Answer from the drawing. Dimensions are ordinates in mm from the lowest x, y and z of the part. A direction names the side the tool comes from. Round coordinates to 2 decimals unless told otherwise and drop trailing zeros. Loops run counter-clockwise (first coordinate to the right, second up) from the corner with the lowest first, then second, coordinate; pieces in that order, holes last. Notation, with made-up numbers: (81.5, 4.5) - (93.5, 4.5) arc R3 cw to (93.5, 9.5) - close; hole circle Ø5 at (50, 0.25). An arc over 180 degrees is marked (long way). Answer as CSV lines item,"result".
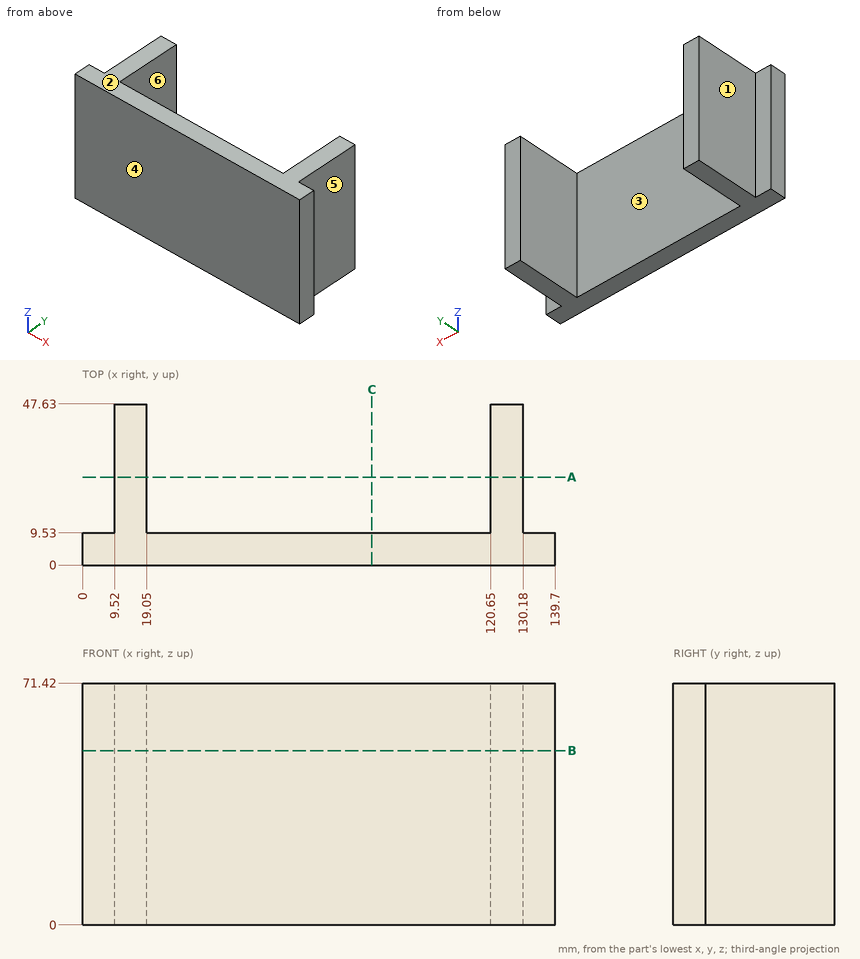
1) A cutting plane is placed at B-B, the plane z = 51.5. Determine the outline of the cut face in (x, y).
Entries:
outline,"(0, 0) - (139.7, 0) - (139.7, 9.53) - (130.18, 9.53) - (130.18, 47.63) - (120.65, 47.63) - (120.65, 9.53) - (19.05, 9.53) - (19.05, 47.63) - (9.52, 47.63) - (9.52, 9.53) - (0, 9.53) - close"
2) The mould has two halves that part along X. Classify the marked faces 1, 2 and 3: pulls with the +X half, pulls with the -X half, needs draft (parallel to the pull), parting line crosses it, or undercut.
Entries:
face 1,"pulls with the -X half"
face 2,"needs draft"
face 3,"undercut"
3) Each of these flat-tipped pins is pushed along its axis until it touches: P1, Ø10, axis at y = 37.5, z = 54.5, coming from the -X side; P2, Ø3, axis at x = 57.5, z = 41.5, coming from the +Y side; P3, Ø19, axis at y = 27, z = 20, coming from the +X side. Where does it stop, or does it pass through?
Entries:
P1,"stops at x = 9.52"
P2,"stops at y = 9.53"
P3,"stops at x = 130.18"
4) A cutting plane is placed at C-C, the plane x = 85.5. Determine the outline of the cut face in (y, z).
Entries:
outline,"(0, 0) - (9.53, 0) - (9.53, 71.42) - (0, 71.42) - close"
5) A tool of negligible diameter and unlimited length cuts with its end or side. For the marked faces 4, 5 and 6, from which of +Z, -Z, +X, -X, +Y, -Y can it reach the whole face along a straight path? Write none if from no direction.
Entries:
face 4,"+Z, -Z, +X, -X, -Y"
face 5,"+Z, -Z, +X, +Y"
face 6,"+Z, -Z, +Y"
6) Find the intervals of material crossed by line 1 (X direction, y = 33, z = 40); line 2 (Y direction, x = 55.5, z = 60.5), in increasing order.
Entries:
line 1,"x = 9.52 to 19.05, 120.65 to 130.18"
line 2,"y = 0 to 9.53"
7) A cutting plane is placed at A-A, the plane y = 26. Determine the outline of the cut face in (x, z), plus the area to 3 significant figures.
Entries:
outline,"(9.52, 0) - (19.05, 0) - (19.05, 71.42) - (9.52, 71.42) - close; (120.65, 0) - (130.18, 0) - (130.18, 71.42) - (120.65, 71.42) - close"
area,"1,360 mm^2"
